Design review of the part built by this model. Coordinates are the model's own, in mm. A direction names the side the tool comes from. Coordinates: 2 decimals unless noted, no trailing zeros. Write each loop counter-clockwise with the first axis right and the second up, starting at its lowest first coordinate (ties: lowest second). Pieces come first, ordered by that corner, then holes. Notation, with made-up numbers: (41, 69) -> (100, 69) arc R23 cw to (100, 83) -> close; hole circle Ø6 at (67, 35.25). An arc over 180 degrees is marked (long way). One line per question, with ' | ' between items. Start each with the question number.
Q1. Add section A-A on x = 0. State the section outline as (y, z) points, and give its area (3 significant figures).
Q2. Draft analysis for pull direction X (two halves, no side actions). For faces 4 (the flat face through (2, 7, 2)), 5 (the cylindrical face through (-1.5, -1.52, 0.07)), 6 (the flat face through (-14, -2, 8)), state which applies: pulls with the +X half, pulls with the -X half, needs draft (parallel to the pull), parting line crosses it, or undercut.
Q3. Add section D-D on y = 6.25. State the section outline as (x, z) points, and give its area (3 significant figures).
Q4. Wall thickness on probe 1 along Z at (x, y) = (0, -1); probe 2 along Z at (x, y) = (0, -4.35); probe 3 along X at (y, z) = (4, 0): over which ranges is each line inside the solid? List them lowest first.
Q5. Add section B-B on y = -0.5. State the section outline as (x, z) points.
Q6. Add section C-C on z = -10.5. State the section outline as (x, y) points.
Q7. For P1, Ø6.5, axis at x = 1.5, z = 1, coming from the -Y side; P2, Ø3.5, axis at x = 0, z = 0, coming from the +Y side; P3, Ø3, axis at y = -3, z = -10.5, coming from the +X side; P4, Ø5.5, axis at x = 0, z = 0, coming from the -Y side, all flat-tipped, find the tip position at first contact; note any pin that passes through.
Q8. For faces 1 (the flat face through (1.3, -3, -1.3)), 2 (the flat face through (0, -2, 15)), 3 (the cylindrical face through (-0.867, 3.958, 3.905)), list the 3-axis set-ups (+Z, -Z, +X, -X, +Y, -Y) from which the entire face can be reached by the end or side of a thin tool; tool diameter is ignored.
from build123d import *

# Parameters (mm, degrees)
PAD_DEPTH       = 5
SKETCH001_R     = 4
SKETCH001_R_2   = 2.4
PAD001_DEPTH    = 7
SKETCH002_R     = 1.5
POCKET_DEPTH    = 12.001
SKETCH003_R     = 3
POCKET001_DEPTH = 2
CHAMFER_SIZE    = 1


with BuildPart() as part:
    # Sketch → Pad (new body)
    with BuildSketch(Plane.XZ):
        with BuildLine():
            Line((-14, 15), (-14, 0))
            ThreePointArc((-14, 0), (0, -14), (14, 0))
            Line((14, 0), (14, 15))
            Line((14, 15), (-14, 15))
        make_face()
    extrude(amount=PAD_DEPTH)

    # Sketch001 (on Face5 of Pad) → Pad001 (join)
    with BuildSketch(Plane(origin=(0, 0, 0), x_dir=(1, 0, 0), z_dir=(0, 1, 0))):
        Circle(SKETCH001_R)
        Circle(SKETCH001_R_2, mode=Mode.SUBTRACT)
    extrude(amount=PAD001_DEPTH)

    # Sketch002 (on Face5 of Pad001) → Pocket (cut, through all)
    with BuildSketch(Plane.XZ.offset(5)):
        Circle(SKETCH002_R)
    extrude(amount=-POCKET_DEPTH, mode=Mode.SUBTRACT)

    # Sketch003 (on Face5 of Pocket) → Pocket001 (cut)
    with BuildSketch(Plane.XZ.offset(5)):
        Circle(SKETCH003_R)
    extrude(amount=-POCKET001_DEPTH, mode=Mode.SUBTRACT)

    # Chamfer
    chamfer_edges = [part.edges().sort_by_distance(p)[0] for p in [
        (-4, 0, 0),
    ]]
    chamfer(chamfer_edges, length=CHAMFER_SIZE)


solid = part.part
Output values:
1) outline: (-5, -14) -> (0, -14) -> (0, -5) -> (1, -4) -> (7, -4) -> (7, -2.4) -> (0, -2.4) -> (0, -1.5) -> (-3, -1.5) -> (-3, -3) -> (-5, -3) -> close; (-5, 3) -> (-3, 3) -> (-3, 1.5) -> (0, 1.5) -> (0, 2.4) -> (7, 2.4) -> (7, 4) -> (1, 4) -> (0, 5) -> (0, 15) -> (-5, 15) -> close | area: 147 mm2
2) face 4: needs draft | face 5: undercut | face 6: pulls with the -X half
3) outline: circle Ø8 at (0, 0); hole circle Ø4.8 at (0, 0) | area: 32.2 mm2
4) probe 1: z = -14 to -1.5, 1.5 to 15 | probe 2: z = -14 to -3, 3 to 15 | probe 3: x = -4 to -2.4, 2.4 to 4
5) outline: (-14, 0) arc R14 ccw to (14, 0) -> (14, 15) -> (-14, 15) -> close; hole circle Ø3 at (0, 0)
6) outline: (-9.26, -5) -> (9.26, -5) -> (9.26, 0) -> (-9.26, 0) -> close
7) P1: stops at y = -5 | P2: stops at y = 0 | P3: stops at x = 10.72 | P4: stops at y = -3
8) face 1: -Y | face 2: +Z, +X, -X, +Y, -Y | face 3: +Y
